Autodesk Inventor part; units mm, degrees
ref_plane "napajeni_znacka2_rovina" through (-1.1, -1.6, -0.4) normal (-1, 0, 0) x (0, 0, 1)
ref_plane "YZ Plane" through (0, 0, 0) normal (1, 0, 0) x (0, 1, 0)
ref_plane "XZ Plane" through (0, 0, 0) normal (0, 1, 0) x (-1, 0, 0)
sketch "Zakladna" plane through (0, 0, 0) normal (0, 0, 1) x (1, 0, 0)
  line L0 (0, 0) -> (78.5, 0)
  line L1 (78.5, 0) -> (78.5, 72)
  line L2 (78.5, 72) -> (0, 72)
  line L3 (0, 72) -> (0, 0)
  dimension "d0" = 78.5
  dimension "d1" = 72
extrude "Extrusion1" add sketch "Zakladna" along normal blind 1.2 and the other way blind 0.4
sketch "Uchyt_arduino" plane through (0, 0, 1.2) normal (0, 0, 1) x (1, 0, 0)
  circle A0 centre (17.2, 60) radius 4
  circle A1 centre (68, 44.8) radius 4
  circle A2 centre (68, 16.9) radius 4
  circle A3 centre (15.9, 11.8) radius 4
  line L0 (0, 72) -> (0, 0)
  dimension "d33" = 8
  dimension "d35" = 8
  dimension "d37" = 8
  dimension "d163" = 17.2
  dimension "d171" = 27.9
  dimension "d173" = 1.3
  dimension "d174" = 50.8
  dimension "d175" = 48.2
  dimension "d176" = 15.2
sketch "Spojeni_srouby" plane through (0, 0, 1.2) normal (0, 0, 1) x (1, 0, 0)
  line L0 (8, 4) -> (8, 0)
  arc A0 (8, 4) -> (4, 8) centre (4, 4) ccw
  line L1 (4, 8) -> (0, 8)
  line L2 (0, 72) -> (0, 0)
  line L3 (0, 8) -> (0, 0)
  line L4 (0, 0) -> (8, 0)
  line L5 (8, 68) -> (8, 72)
  arc A1 (4, 64) -> (8, 68) centre (4, 68) ccw
  line L6 (4, 64) -> (0, 64)
  line L7 (0, 0) -> (0, 72)
  line L8 (0, 64) -> (0, 72)
  line L9 (0, 72) -> (8, 72)
  line L10 (70.5, 4) -> (70.5, 0)
  arc A2 (74.5, 8) -> (70.5, 4) centre (74.5, 4) ccw
  line L11 (74.5, 8) -> (78.5, 8)
  line L12 (78.5, 8) -> (78.5, 0)
  line L13 (78.5, 0) -> (70.5, 0)
  line L14 (70.5, 68) -> (70.5, 72)
  arc A3 (70.5, 68) -> (74.5, 64) centre (74.5, 68) ccw
  line L15 (74.5, 64) -> (78.5, 64)
  line L16 (78.5, 64) -> (78.5, 72)
  line L17 (78.5, 72) -> (70.5, 72)
  line L18 (78.5, 0) -> (78.5, 72)
extrude "Extrusion2" add sketch "Uchyt_arduino" along normal blind 7
extrude "Extrusion5" add sketch "Spojeni_srouby" along normal blind 15
sketch "diry_srouby" plane through (0, 0, 16.2) normal (0, 0, 1) x (1, 0, 0)
  arc A0 (8, 4) -> (4, 8) centre (4, 4) ccw
  arc A1 (74.5, 8) -> (70.5, 4) centre (74.5, 4) ccw
  arc A2 (70.5, 68) -> (74.5, 64) centre (74.5, 68) ccw
  arc A3 (4, 64) -> (8, 68) centre (4, 68) ccw
  point P0 (0, 0)
hole "Hole6" at (4, 4, 16.2) at (74.5, 4, 16.2) at (74.5, 68, 16.2) at (4, 68, 16.2) direction (0, 0, -1) diameter 2.8 end through all
sketch "steny" plane through (0, 0, 1.2) normal (0, 0, 1) x (1, 0, 0)
  line L0 (0, 72) -> (0, 56.55)
  line L1 (0, 56.55) -> (-1.6, 56.55)
  line L2 (-1.6, 56.55) -> (-1.6, 72)
  line L3 (-1.6, 72) -> (-1.6, 73.6)
  line L4 (-1.6, 73.6) -> (80.1, 73.6)
  line L5 (80.1, 73.6) -> (80.1, 0)
  line L6 (80.1, 0) -> (80.1, -1.6)
  line L7 (80.1, -1.6) -> (0, -1.6)
  line L8 (0, -1.6) -> (-1.6, -1.6)
  line L9 (-1.6, -1.6) -> (-1.6, 39.75)
  line L10 (-1.6, 39.75) -> (0, 39.75)
  line L11 (0, 0) -> (0, 72)
  line L12 (0, 39.75) -> (0, 0)
  line L13 (0, 0) -> (78.5, 0)
  line L14 (8, 0) -> (78.5, 0)
  line L15 (78.5, 0) -> (0, 0)
  line L16 (78.5, 0) -> (0, 0)
  line L17 (78.5, 72) -> (78.5, 0)
  line L18 (0, 0) -> (78.5, 0)
  line L19 (78.5, 0) -> (78.5, 72)
  line L20 (0, 72) -> (78.5, 72)
  line L21 (78.5, 72) -> (0, 72)
  line L22 (92, 0) -> (92, 8)
  point P0 (78.5, 0)
  point P1 (78.5, 8)
  dimension "d133" = 15.45
  dimension "d134" = 1.6
  dimension "d135" = 1.6
  dimension "d137" = 1.6
  dimension "d138" = 1.6
  dimension "d139" = 16.8
  dimension "d179" = 1.6
extrude "Extrusion6" add sketch "steny" along normal blind 31.5 and the other way blind 1.6 contours L0 L1 L2 L3 L4 L5 L6 L7 L8 L9 L10 L11 L13 L17 L20
sketch "stena_RJ45" plane through (0, 0, 1.2) normal (0, 0, 1) x (1, 0, 0)
  line L0 (-1.6, 56.55) -> (0, 56.55)
  line L1 (0, 39.75) -> (-1.6, 39.75)
  line L2 (-1.6, 39.75) -> (0, 39.75)
  line L3 (0, 56.55) -> (0, 39.75)
  line L4 (0, 56.55) -> (0, 39.75)
  line L5 (0, 56.55) -> (-1.6, 56.55)
  line L6 (-1.6, 56.55) -> (-1.6, 39.75)
  line L7 (0, 39.75) -> (-1.6, 39.75)
  point P0 (0, 0)
extrude "Extrusion7" add sketch "stena_RJ45" along normal blind 10.9 and the other way blind 1.6
sketch "arduino_uchyt_zavitovaVlozka" plane through (17.2, 60, 8.2) normal (0, 0, 1) x (1, 0, 0)
  circle A0 centre (50.8, -43.1) radius 4
  circle A1 centre (50.8, -15.2) radius 4
  circle A2 centre (0, 0) radius 4
  circle A3 centre (-1.3, -48.2) radius 4
  point P0 (-17.2, -60)
hole "Hole7" at (68, 16.9, 8.2) at (68, 44.8, 8.2) at (17.2, 60, 8.2) at (15.9, 11.8, 8.2) direction (0, 0, -1) diameter 3.3 depth 7 countersink diameter 3.75 countersink angle 10
sketch "napajeni_znacka1" plane through (-1.6, -1.6, -0.4) normal (-1, 0, 0) x (0, 0, 1)
  circle A0 centre (20.1, 31.85) radius 0.4
  line L0 (12.5, 41.35) -> (33.1, 41.35)
  line L1 (0, 0) -> (0, 75.2)
  point P0 (0.4, 1.6)
  dimension "d155" = 0.8
  dimension "d156" = 9.5
  dimension "d157" = 20.1
ref_plane "napajeni_znacka2_rovina" through (-1.1, -1.6, -0.4) normal (-1, 0, 0) x (0, 0, 1)
sketch "napajeni_znacka2" plane through (-1.1, -1.6, -0.4) normal (-1, 0, 0) x (0, 0, 1)
  point P0 (0.4, 1.6)
  point P1 (20.1, 31.85)
  point P2 (20.1, 31.85)
loft "Loft4" cut profiles "napajeni_znacka1" section 2 point at (-1.1, 30.25, 19.7)
sketch "vyrez_nepouzity_jack" plane through (0, 8, 1.2) normal (1, 0, 0) x (0, 0, -1)
  line L0 (-8, 15.35) -> (-33, 15.35)
  line L1 (-33, 15.35) -> (-33, 3.35)
  line L2 (-33, 3.35) -> (-8, 3.35)
  line L3 (-8, 3.35) -> (-8, 15.35)
  line L4 (-10.9, 31.75) -> (-31.5, 31.75)
  line L5 (0, 56) -> (0, 0)
  point P0 (1.2, -8)
  dimension "d164" = 25
  dimension "d165" = 12
  dimension "d166" = 16.4
  dimension "d167" = 8
extrude "Extrusion8" cut sketch "vyrez_nepouzity_jack" against normal blind 0.5
fillet "Fillet1" radius 2 4 edges at (-1.6, -1.6, 16.15) (80.1, -1.6, 16.15) (-1.6, 73.6, 16.15) (80.1, 73.6, 16.15)
properties part number "case_bottom"
Source: CAD feature listing. Evaluate the final solid. Frame: model axes, mm. A direction names the side the tool comes from. Round coordinates to 2 decimals unless told otherwise and drop trailing zeros. Order: outer loops, then holes, each group sorted by start corner. A loop starts at its lowest first (then second) coordinate and runs counter-clockwise, first axis right, second up. Notation, with made-up numbers: (-3.5, 38) -> (46.5, 38) arc R22 cw to (46.5, 51) -> close; hole circle Ø4 at (20.5, 29.25). An arc over 180 degrees is marked (long way). One line per item, written item: value. Start each with the question number.
Q1. Draft query along Y for faces 3 (the flat face through (76, 8, 9)), 4 (the cylindrical face through (79.53, -1, 15.92)), 5 (the cylindrical face through (-1.03, 73, 15.92)). Return one class per face: pulls with the +Y half, pulls with the -Y half, needs draft (parallel to the pull), parting line crosses it, or undercut.
Q2. Section query B-B (y = 38.5). Return the cut outline in (x, z).
Q3. Section query D-D (x = 48.5). Return the cut outline in (y, z), plus the area to 3 significant figures.
Q4. Access query for faces 1 (the cylindrical face through (75.74, 67.35, 7.78)), 2 (the cylindrical face through (71.703, 65.141, 8.595)). Directions: +Z, -Z, +X, -X, +Y, -Y. A direction counts if a zero-diameter tool reaches every point of the face in a straight line with its end or side. Return the directions, or none.
Q5. Section query C-C (z = 26). Return the cut outline in (x, y), plus the area to 3 significant figures.
Q6. Material intervals for probe 1 along X at (y, z) = (68, 7.25); probe 2 along Y at (x, z) = (68, 2.9); probe 3 along Y at (x, z) = (74.5, 8), sorted ascending.
Q7. Section query A-A (z = 4). Give the number of separate pieces and of enclosed holes in the cut face, plus the area to 3 significant figures.
Q8. Pin query (flat end, axial travel): pin 1 (2.5 mm diameter, centred on x = 74.5, y = 4, fed in from -Z); pin 2 (9 mm diameter, centred on x = 18.5, y = 59, fed in from +Z); pin 3 (2.5 mm diameter, centred on x = 68, y = 44.8, fed in from +Z); pin 4 (3 mm diameter, centred on x = 4, y = 4, fed in from +Z). Return the tip coordinate at first contact, or that it passes through.
Findings below:
1. face 3: undercut
1. face 4: pulls with the -Y half
1. face 5: pulls with the +Y half
2. outline: (-1.6, -0.4) -> (80.1, -0.4) -> (80.1, 32.7) -> (78.5, 32.7) -> (78.5, 1.2) -> (0, 1.2) -> (0, 32.7) -> (-1.6, 32.7) -> close
3. outline: (-1.6, -0.4) -> (73.6, -0.4) -> (73.6, 32.7) -> (72, 32.7) -> (72, 1.2) -> (0, 1.2) -> (0, 32.7) -> (-1.6, 32.7) -> close
3. area: 221 mm²
4. face 1: +Z, -Z
4. face 2: +Z
5. outline: (-1.6, 0.4) arc R2 ccw to (0.4, -1.6) -> (78.1, -1.6) arc R2 ccw to (80.1, 0.4) -> (80.1, 71.6) arc R2 ccw to (78.1, 73.6) -> (0.4, 73.6) arc R2 ccw to (-1.6, 71.6) -> (-1.6, 56.55) -> (0, 56.55) -> (0, 72) -> (78.5, 72) -> (78.5, 0) -> (0, 0) -> (0, 11.35) -> (-0.5, 11.35) -> (-0.5, 23.35) -> (0, 23.35) -> (0, 39.75) -> (-1.6, 39.75) -> close
5. area: 456 mm²
6. probe 1: -1.6 to 2.6, 5.4 to 8, 70.5 to 73.1, 75.9 to 80.1
6. probe 2: -1.6 to 0, 12.9 to 15.25, 18.55 to 20.9, 40.8 to 43.15, 46.45 to 48.8, 72 to 73.6
6. probe 3: -1.6 to 2.6, 5.4 to 8, 64 to 66.6, 69.4 to 73.6
7. separate pieces: 5
7. enclosed holes: 9
7. area: 873 mm²
8. pin 1: through
8. pin 2: z = 8.2
8. pin 3: z = 1.2
8. pin 4: z = 16.2
